```python
from build123d import *

# Parameters (mm, degrees)
F1_DEPTH  = 50.8
F2_W      = 15.24
F2_H      = 30.48
F3_DEPTH  = 63.5
F4_W      = 15.24
F4_H      = 30.48
F5_DEPTH  = 63.5
F7_DEPTH  = 38.1
F9_DEPTH  = 38.1
F11_DEPTH = 38.1
F10_W     = 3.175
F10_H     = 3.175
F12_DEPTH = 38.1
F15_DEPTH = 0.254


with BuildPart() as f1:
    # F0 (on Front) → F1 (new body)
    with BuildSketch(Plane.XZ):
        Polygon((-12.7, 0), (0, 0), (12.7, 0), (12.7, 31.75), (0, 50.8), (-12.7, 31.75), align=None)
    extrude(amount=F1_DEPTH)

    # F2 (on Top) → F3 (join)
    with BuildSketch(Plane.XY):
        with Locations((-7.62, 15.24)):
            Rectangle(F2_W, F2_H)
    extrude(amount=F3_DEPTH)

    # F4 (on Top) → F5 (join)
    with BuildSketch(Plane.XY):
        with Locations((7.62, 15.24)):
            Rectangle(F4_W, F4_H)
    extrude(amount=F5_DEPTH)

    # F6 (on face) → F7 (join)
    with BuildSketch(Plane.YZ.offset(15.24)):
        Polygon((2.54, 0), (15.24, 0), (27.94, 0), (27.94, 31.75), (15.24, 50.8), (2.54, 31.75), align=None)
    extrude(amount=F7_DEPTH)

    # F8 (on face) → F9 (join)
    with BuildSketch(Plane(origin=(-15.24, 0, 0), x_dir=(0, -1, 0), z_dir=(-1, 0, 0))):
        Polygon((-27.94, 0), (-15.24, 0), (-2.54, 0), (-2.54, 31.75), (-15.24, 50.8), (-27.94, 31.75), align=None)
    extrude(amount=F9_DEPTH)

    # F10 (on face) → F11 (join)
    with BuildSketch(Plane(origin=(0, 0, 0), x_dir=(1, 0, 0), z_dir=(0, 0, -1))):
        Polygon((9.525, 50.8), (12.7, 50.8), (15.875, 50.8), (15.875, 53.975), (9.525, 53.975), align=None)
    extrude(amount=-F11_DEPTH)

    # F10 (on face) → F12 (join)
    with BuildSketch(Plane(origin=(0, 0, 0), x_dir=(1, 0, 0), z_dir=(0, 0, -1))):
        Polygon((9.525, 50.8), (12.7, 50.8), (15.875, 50.8), (15.875, 53.975), (9.525, 53.975), align=None)
        with Locations((14.2875, 49.2125)):
            Rectangle(F10_W, F10_H)
        with Locations((11.1125, 49.2125)):
            Rectangle(F10_W, F10_H)
        with Locations((-14.2875, 49.2125)):
            Rectangle(F10_W, F10_H)
        with Locations((-11.1125, 49.2125)):
            Rectangle(F10_W, F10_H)
        Polygon((-15.875, 50.8), (-12.7, 50.8), (-9.525, 50.8), (-9.525, 53.975), (-15.875, 53.975), align=None)
    extrude(amount=-F12_DEPTH)

    # F13 (on face) → F15 (join)
    with BuildSketch(Plane.XZ.offset(50.8)):
        with BuildLine():
            Line((-1.905, 0), (0, 0))
            Line((0, 0), (0, 6.35))
            ThreePointArc((0, 6.35), (-1.392212, 5.026327), (-1.905, 3.175))
            Line((-1.905, 3.175), (-1.905, 0))
        make_face()
        with BuildLine():
            Line((0, 6.35), (0, 0))
            Line((0, 0), (1.905, 0))
            Line((1.905, 0), (1.905, 3.175))
            ThreePointArc((1.905, 3.175), (1.392212, 5.026327), (0, 6.35))
        make_face()
    extrude(amount=F15_DEPTH)


solid = f1.part
```
Build history of the part. All positions in model axes, mm. A direction names the side the tool comes from. Round coordinates to 2 decimals unless told otherwise and drop trailing zeros. Write each loop counter-clockwise with the first axis right and the second up, starting at its lowest first coordinate (ties: lowest second). Pieces come first, ordered by that corner, then holes.
1) Band-saw the part on C-C, the plane y = 24. List the corners of the cut face in (x, z).
2) Band-saw the part on A-A, the plane z = 41.5. List the corners of the cut face in (x, y), and give its area (3 significant figures).
3) 3-axis set-ups, long thin cutter, end or side, ignore diameter. For faces 4 (the flat face through (34.02, 21.68, 41.14)), 5 (the flat face through (-15.875, -51, 19)), 6 (the flat face through (-15.24, 8, 45)), 7 (the flat face through (-13, -51, 38.1)): which of +Z, -Z, +X, -X, +Y, -Y reach the whole face in a straight line?
4) Mould opens along X. For faces 1 (the flat face through (0, -51.054, 3)), 2 (the flat face through (-53.34, 15, 20)), 3 (the flat face through (-14, -47.625, 19)) say: +X half, -X half, draft (parallel to the pull), parting line (faces both ways), or undercut.
5) Band-saw the part on D-D, the plane z = 9.5. List the corners of the cut face in (x, y) (3 decimals).
6) Pin check, flat tips, straight feed: pin 1 (12 mm diameter, centred on y = -41, z = 17, fed in from +X); pin 2 (1.9 mm diameter, centred on y = -50, z = 25.5, fed in from -X) (3 decimals); pin 3 (15 mm diameter, centred on x = -1.5, z = 22.5, fed in from -Y). Stop position of each tip, or through.
7) Band-saw the part on B-B, the plane x = -5. List the corners of the cut face in (y, z), and give its area (3 significant figures).
8) Drill centre lines: probe 1 along X at (y, z) = (-21.5, 27); probe 2 along X at (y, z) = (18, 56.5); probe 3 along Y at (x, z) = (30, 26). Where is each one in solid material? Low to high.
Ans:
1. outline: (-53.34, 0) - (53.34, 0) - (53.34, 37.66) - (15.24, 37.66) - (15.24, 63.5) - (-15.24, 63.5) - (-15.24, 37.66) - (-53.34, 37.66) - close
2. outline: (-53.34, 9.04) - (-15.24, 9.04) - (-15.24, 0) - (-6.2, 0) - (-6.2, -50.8) - (6.2, -50.8) - (6.2, 0) - (15.24, 0) - (15.24, 9.04) - (53.34, 9.04) - (53.34, 21.44) - (15.24, 21.44) - (15.24, 30.48) - (-15.24, 30.48) - (-15.24, 21.44) - (-53.34, 21.44) - close
2. area: 2,500 mm2
3. face 4: +Z, +X, +Y
3. face 5: +Z, -Z, -X, -Y
3. face 6: +Z, -X
3. face 7: +Z, -X, -Y
4. face 1: undercut
4. face 2: -X half
4. face 3: draft
5. outline: (-53.34, 2.54) - (-15.24, 2.54) - (-15.24, 0) - (-12.7, 0) - (-12.7, -47.625) - (-15.875, -47.625) - (-15.875, -53.975) - (-9.525, -53.975) - (-9.525, -50.8) - (9.525, -50.8) - (9.525, -53.975) - (15.875, -53.975) - (15.875, -47.625) - (12.7, -47.625) - (12.7, 0) - (15.24, 0) - (15.24, 2.54) - (53.34, 2.54) - (53.34, 27.94) - (15.24, 27.94) - (15.24, 30.48) - (-15.24, 30.48) - (-15.24, 27.94) - (-53.34, 27.94) - close
6. pin 1: stops at x = 12.7
6. pin 2: stops at x = -15.875
6. pin 3: stops at y = -50.8
7. outline: (-50.8, 0) - (30.48, 0) - (30.48, 63.5) - (0, 63.5) - (0, 43.3) - (-50.8, 43.3) - close
7. area: 4,140 mm2
8. probe 1: x = -12.7 to 12.7
8. probe 2: x = -15.24 to 15.24
8. probe 3: y = 2.54 to 27.94
